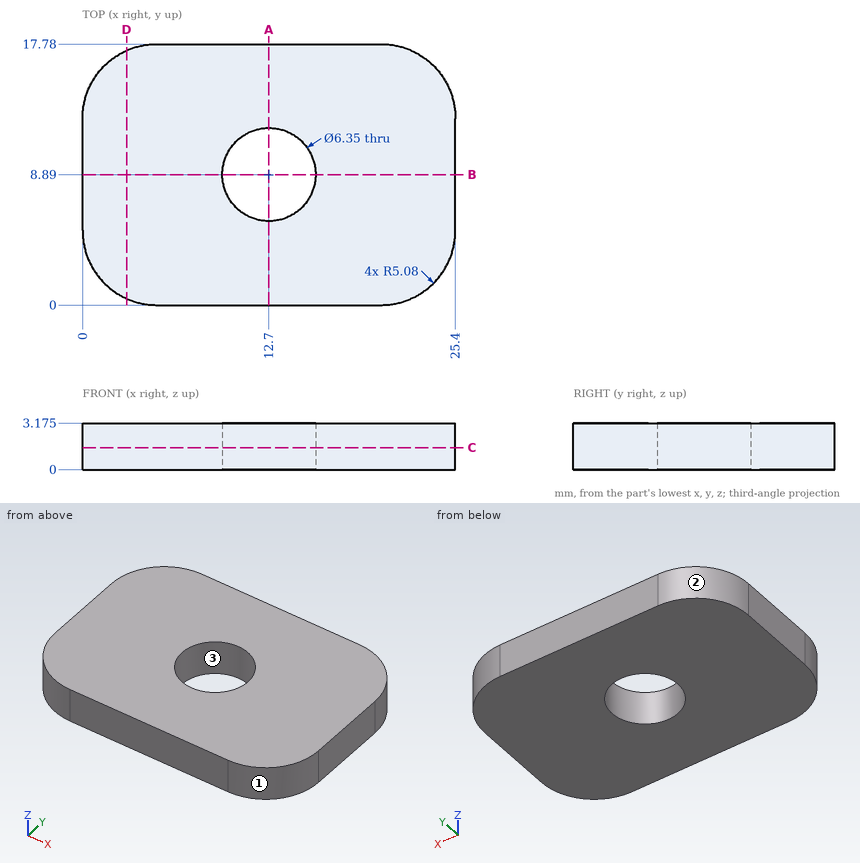
Answer from the drawing. Dimensions are ordinates in mm from the lowest x, y and z of the part. Round coordinates to 2 decimals unless told otherwise and drop trailing zeros. Order: outer loops, then holes, each group sorted by start corner. A loop starts at its lowest first (then second) coordinate and runs counter-clockwise, first axis right, second up. Notation, with made-up numbers: (80, 39) - (134, 39) arc R24 ccw to (134, 67) - close; hole circle Ø5 at (-6.75, 18.25). An arc over 180 degrees is marked (long way). Put each result on its own line as item: value. Start each with the question number.
(1) Given P1, Ø1.5, axis at x = 3.5, z = 2, coming from the -Y side, flat-ended and moving along its own axis, determine where the tip first touches the part or whether it passes through.
(2) Find section B-B (y = 8.89). Give the vertices of the cut face in (x, z) (3 decimals).
(3) Find section A-A (x = 12.7). Give the vertices of the cut face in (y, z) (3 decimals), plus the area to 3 significant figures.
(4) Determine the mould class of the marked faces 1, 2 and 3 for opening direction Y: released by +Y, released by -Y, zero draft, split by the parting line, or undercut.
(5) Straight lines are drawn through the part: probe 1 along Y at (x, z) = (12.7, 2.45) (3 decimals); probe 2 along Y at (x, z) = (5, 1.05); probe 3 along Y at (x, z) = (15.5, 2.25). For each, find the intervals that lie inside material, in ascending order. Write a range as from..to.
(6) Find section C-C (z = 1.5). Give the vertices of the cut face in (x, y) (3 decimals), plus the area to 3 significant figures.
(7) Find section D-D (x = 3). Give the vertices of the cut face in (y, z) (3 decimals).
Reply:
1. P1: y = 0.07
2. outline: (0, 0) - (9.525, 0) - (9.525, 3.175) - (0, 3.175) - close; (15.875, 0) - (25.4, 0) - (25.4, 3.175) - (15.875, 3.175) - close
3. outline: (0, 0) - (5.715, 0) - (5.715, 3.175) - (0, 3.175) - close; (12.065, 0) - (17.78, 0) - (17.78, 3.175) - (12.065, 3.175) - close
3. area: 36.3 mm^2
4. face 1: released by -Y
4. face 2: released by +Y
4. face 3: undercut
5. probe 1: 0..5.715, 12.065..17.78
5. probe 2: 0..17.78
5. probe 3: 0..7.39, 10.39..17.78
6. outline: (0, 5.08) arc R5.08 ccw to (5.08, 0) - (20.32, 0) arc R5.08 ccw to (25.4, 5.08) - (25.4, 12.7) arc R5.08 ccw to (20.32, 17.78) - (5.08, 17.78) arc R5.08 ccw to (0, 12.7) - close; hole circle Ø6.35 at (12.7, 8.89)
6. area: 398 mm^2
7. outline: (0.445, 0) - (17.335, 0) - (17.335, 3.175) - (0.445, 3.175) - close
